Work out the finished part from the listing and answer in its coordinate system (mm). Round coordinates to 2 decimals unless told otherwise and drop trailing zeros. Order: outer loops, then holes, each group sorted by start corner. A loop starts at its lowest first (then second) coordinate and runs counter-clockwise, first axis right, second up. Notation, with made-up numbers: M 34,41 L 47,41 A22 cw 47,68 Z; hole C 36,33.5 d10. An arc over 180 degrees is marked long. Return JSON: item names as keys, results as strings.
from build123d import *

# Parameters (mm, degrees)
SKETCH1_W            = 44.45
SKETCH1_H            = 15.875
BOSS_EXTRUDE1_DEPTH  = 3.175
M4_CLEARANCE_HOLE1_D = 4.5
FILLET1_R            = 3.175


with BuildPart() as part:
    # Sketch1 → Boss-Extrude1 (new body)
    with BuildSketch(Plane.XY):
        Rectangle(SKETCH1_W, SKETCH1_H)
    extrude(amount=BOSS_EXTRUDE1_DEPTH)

    # M4 Clearance Hole1 (through all)
    with Locations(Plane(origin=(0, 0, 0), x_dir=(-1, 0, 0), z_dir=(0, 0, -1))):
        with Locations((-14.2875, 0), (14.2875, 0)):
            Hole(M4_CLEARANCE_HOLE1_D / 2)

    # Fillet1
    fillet1_edges = [part.edges().sort_by_distance(p)[0] for p in [
        (22.225, -7.9375, 1.5875),
        (-22.225, -7.9375, 1.5875),
        (-22.225, 7.9375, 1.5875),
        (22.225, 7.9375, 1.5875),
    ]]
    fillet(fillet1_edges, radius=FILLET1_R)


solid = part.part
Item 1: Find section C-C (x = -16). Determine the outline of the cut face in (y, z) (1 decimal).
Output:
{"outline": "M -7.9,0 L -1.5,0 L -1.5,3.2 L -7.9,3.2 Z; M 1.5,0 L 7.9,0 L 7.9,3.2 L 1.5,3.2 Z"}
Item 2: The mould has two halves that part along Y. Classify faces 1 (the flat face through (-22.225, 0, 2)), 2 (the cylindrical face through (-16.535, 0.099, 1.61)), 3 (the cylindrical face through (-21.3, 7, 1.6)), 4 (the cylindrical face through (16.434, 0.676, 1.61)): pulls with the +Y half, pulls with the -Y half, needs draft (parallel to the pull), parting line crosses it, or undercut.
Output:
{"face 1": "needs draft", "face 2": "undercut", "face 3": "pulls with the +Y half", "face 4": "undercut"}
Item 3: Find section B-B (z = 1.95). State how many separate pieces and enclosed holes the cut face has, plus the area to 3 significant figures.
Output:
{"separate pieces": "1", "enclosed holes": "2", "area": "665 mm^2"}
Item 4: Find section A-A (y = 0). Determine the outline of the cut face in (x, z) (1 decimal), plus the area to 3 significant figures.
Output:
{"outline": "M -22.2,0 L -16.5,0 L -16.5,3.2 L -22.2,3.2 Z; M -12,0 L 12,0 L 12,3.2 L -12,3.2 Z; M 16.5,0 L 22.2,0 L 22.2,3.2 L 16.5,3.2 Z", "area": "113 mm^2"}
Item 5: Find section D-D (y = 1.75). Determine the outline of the cut face in (x, z) (3 decimals), plus the area to 3 significant figures.
Output:
{"outline": "M -22.225,0 L -15.702,0 L -15.702,3.175 L -22.225,3.175 Z; M -12.873,0 L 12.873,0 L 12.873,3.175 L -12.873,3.175 Z; M 15.702,0 L 22.225,0 L 22.225,3.175 L 15.702,3.175 Z", "area": "123 mm^2"}
Item 6: Consider line 1 along X through (y, z) = (1, 1.9) (3 decimals); line 2 along X through (y, z) = (-1.25, 0.95) (3 decimals); line 3 along X through (y, z) = (-5, 2.95). Determine where each line is inside the solid, lowest interval first. Write a range as [from, to].
Output:
{"line 1": "x = [-22.225, -16.303], [-12.272, 12.272], [16.303, 22.225]", "line 2": "x = [-22.225, -16.158], [-12.417, 12.417], [16.158, 22.225]", "line 3": "x = [-22.22, 22.22]"}
